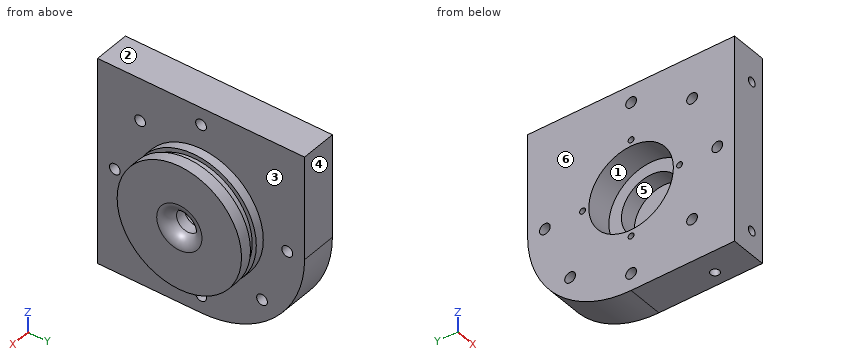
```python
from build123d import *

# Parameters (mm, degrees)
SKETCH1_R                     = 36.6395
HOUSING_FITTING_EXTRUDE_DEPTH = 16.637
HOUSING_BODY_1_DEPTH          = 21.2852
SKETCH3_R                     = 6.731
IMPELLER_BORE_DEPTH           = 17.018
SKETCH4_R                     = 4
SHAFT_BORE_DEPTH              = 20.9042
O_RING_CUT_DEPTH              = 1.27
O_RING_CUT_DEPTH_BACK         = 3.175
SKETCH5_R                     = 36.6395
SKETCH5_R_2                   = 34.2265
SKETCH12_R                    = 3.175
CUT_EXTRUDE2_DEPTH            = 21.2852
CIRPATTERN1_COUNT             = 8
SKETCH14_R                    = 2.5796875
CUT_EXTRUDE4_DEPTH            = 16.51
SKETCH15_R                    = 2.5796875
CUT_EXTRUDE5_DEPTH            = 10.922
FILLET1_R                     = 6.604
SKETCH17_R                    = 17.5006
CUT_EXTRUDE8_DEPTH            = 25.2222
SKETCH18_R                    = 24.9174
CUT_EXTRUDE9_DEPTH            = 15.3162
SKETCH19_R                    = 1.7272
CUT_EXTRUDE10_DEPTH           = 9.525


with BuildPart() as part:
    # Sketch1 → Housing Fitting Extrude (new body)
    with BuildSketch(Plane(origin=(0, 0, 0), x_dir=(0, 0, -1), z_dir=(1, 0, 0))):
        Circle(SKETCH1_R)
    extrude(amount=HOUSING_FITTING_EXTRUDE_DEPTH)

    # Sketch2 → Housing Body 1 (add)
    with BuildSketch(Plane.ZY):
        with BuildLine():
            Line((60.96, 0), (60.96, 60.96))
            Line((60.96, 60.96), (0, 60.96))
            ThreePointArc((0, 60.96), (-43.105229381, 43.105229381), (-60.96, 0))
            Line((-60.96, 0), (-60.96, -54.61))
            Line((-60.96, -54.61), (-60.96, -60.96))
            Line((-60.96, -60.96), (60.96, -60.96))
            Line((60.96, -60.96), (60.96, -54.61))
            Line((60.96, -54.61), (60.96, 0))
        make_face()
    extrude(amount=HOUSING_BODY_1_DEPTH)

    # Sketch3 → Impeller Bore (cut)
    with BuildSketch(Plane(origin=(16.637, 0, 0), x_dir=(0, 0, -1), z_dir=(1, 0, 0))):
        Circle(SKETCH3_R)
    extrude(amount=-IMPELLER_BORE_DEPTH, mode=Mode.SUBTRACT)

    # Sketch4 → Shaft Bore (cut)
    with BuildSketch(Plane(origin=(-0.381, 0, 0), x_dir=(0, 0, -1), z_dir=(1, 0, 0))):
        Circle(SKETCH4_R)
    extrude(amount=-SHAFT_BORE_DEPTH, mode=Mode.SUBTRACT)

    # Sketch5 → O-Ring Cut (cut, two sides: drawn at the far end of the back side and taken through both)
    with BuildSketch(Plane(origin=(8.509, 0, 0), x_dir=(0, 0, -1), z_dir=(1, 0, 0)).offset(-O_RING_CUT_DEPTH_BACK)):
        Circle(SKETCH5_R)
        Circle(SKETCH5_R_2, mode=Mode.SUBTRACT)
    extrude(amount=O_RING_CUT_DEPTH + O_RING_CUT_DEPTH_BACK, mode=Mode.SUBTRACT)

    # Sketch12 → Cut-Extrude2 (cut)
    with BuildSketch(Plane(origin=(0, 0, 0), x_dir=(0, 0, -1), z_dir=(1, 0, 0))):
        with Locations((-50.8, 0)):
            Circle(SKETCH12_R)
    cut_extrude2 = extrude(amount=-CUT_EXTRUDE2_DEPTH, mode=Mode.SUBTRACT)

    # CirPattern1: Cut-Extrude2 ×8 about axis, 1 skipped
    cirpattern1_axis = Axis((0, 0, 0), (1, 0, 0))
    add([cut_extrude2.rotate(cirpattern1_axis, i * 360 / CIRPATTERN1_COUNT) for i in range(1, CIRPATTERN1_COUNT) if i not in (7,)], mode=Mode.SUBTRACT)

    # Sketch14 → Cut-Extrude4 (cut)
    with BuildSketch(Plane.XZ.offset(60.96)):
        with Locations(Location((-8.128, -46.754349092, 0), (0, 0, 270))):
            Circle(SKETCH14_R)
        with Locations(Location((-8.128, 41.914080666, 0), (0, 0, 270))):
            Circle(SKETCH14_R)
    extrude(amount=-CUT_EXTRUDE4_DEPTH, mode=Mode.SUBTRACT)

    # Sketch15 → Cut-Extrude5 (cut)
    with BuildSketch(Plane(origin=(0, 0, -60.96), x_dir=(-1, 0, 0), z_dir=(0, 0, -1))):
        with Locations(Location((8.128, -39.337514031, 0), (0, 0, 90))):
            Circle(SKETCH15_R)
    extrude(amount=-CUT_EXTRUDE5_DEPTH, mode=Mode.SUBTRACT)

    # Fillet1
    fillet1_edges = [part.edges().sort_by_distance(p)[0] for p in [
        (16.637, 0, 6.731),
    ]]
    fillet(fillet1_edges, radius=FILLET1_R)

    # Sketch17 → Cut-Extrude8 (cut)
    with BuildSketch(Plane.ZY.offset(21.2852)):
        Circle(SKETCH17_R)
    extrude(amount=-CUT_EXTRUDE8_DEPTH, mode=Mode.SUBTRACT)

    # Sketch18 → Cut-Extrude9 (cut)
    with BuildSketch(Plane.ZY.offset(21.2852)):
        Circle(SKETCH18_R)
    extrude(amount=-CUT_EXTRUDE9_DEPTH, mode=Mode.SUBTRACT)

    # Sketch19 → Cut-Extrude10 (cut)
    with BuildSketch(Plane.ZY.offset(21.2852)):
        with Locations((0, 28.575)):
            Circle(SKETCH19_R)
        with Locations((28.575, 0)):
            Circle(SKETCH19_R)
        with Locations((0, -28.575)):
            Circle(SKETCH19_R)
        with Locations((-28.575, 0)):
            Circle(SKETCH19_R)
    extrude(amount=-CUT_EXTRUDE10_DEPTH, mode=Mode.SUBTRACT)


solid = part.part
```
Geometry: final body of the model. Coordinates: model frame, mm. Face numbers are marked on the shaded views. A direction names the side the tool comes from. Round coordinates to 2 decimals unless told otherwise and drop trailing zeros. Order: outer loops, then holes, each group sorted by start corner. A loop starts at its lowest first (then second) coordinate and runs counter-clockwise, first axis right, second up. Notation, with made-up numbers: M 37,-6.5 L 86,-6.5 A11 ccw 86,7.5 Z; hole C 89,84.25 d10. An arc over 180 degrees is marked long. Use one line per item in the form item = value. Start each with the question number.
Q1. Material intervals for line 1 (Y direction, x = 6.25, z = 0); line 2 (Y direction, x = -9, z = 50.5); line 3 (Y direction, x = -13.5, z = 2), sorted ascending. Write a range as [from, to].
Q2. Pin query (flat end, axial travel): pin 1 Ø2 at (x, y) = (10.5, -26) entering from +Z; pin 2 Ø1.5 at (y, z) = (-29, -27) entering from +X; pin 3 Ø21.5 at (y, z) = (0, 0) entering from +X. Return the tip coordinate at first contact, or that it passes through.
Q3. Cut plane A-A (z = 50.8). Return loops of the section in (x, y) (3 decimals).
Q4. Cut plane C-C (y = 50.8). Return loops of the section in (x, z) (3 decimals).
Q5. Access query for the marked faces 1, 2 and 3. Directions: +Z, -Z, +X, -X, +Y, -Y. A direction counts if a zero-diameter tool reaches every point of the face in a straight line with its end or side. Return the directions, or none.
Q6. Cut plane B-B (y = -49.5). Return loops of the section in (x, z), and give its area (3 significant figures).
Q7. Cut plane D-D (y = 22). Return loops of the section in (x, z), and give its area (3 significant figures).
Q8. Mould query, pull axis Y, two halves, no side actions, for the marked faces 4, 5 and 6. Classes: +Y half, -Y half, draft (parallel to the pull), parting line (faces both ways), or undercut.
Geometry results:
q1.line_1 = [-34.23, -6.73], [6.73, 34.23]
q1.line_2 = [-60.96, -3.16], [3.16, 60.96]
q1.line_3 = [-60.96, -53.27], [-48.33, -24.84], [24.84, 48.33], [53.27, 60.96]
q2.pin_1 = 26.79
q2.pin_2 = 0
q2.pin_3 = 16.11
q3.outline = M -21.285,-60.96 L 0,-60.96 L 0,-3.175 L -21.285,-3.175 Z; M -21.285,3.175 L 0,3.175 L 0,60.96 L -21.285,60.96 Z
q4.outline = M -21.285,-33.697 L 0,-33.697 L 0,-3.175 L -21.285,-3.175 Z; M -21.285,3.175 L 0,3.175 L 0,60.96 L -21.285,60.96 Z
q5.face_1 = -X
q5.face_2 = +Z, +X, -X, +Y, -Y
q5.face_3 = +X
q6.outline = M -21.29,-60.96 L 0,-60.96 L 0,-2.9 L -21.29,-2.9 Z; M -21.29,2.9 L 0,2.9 L 0,60.96 L -21.29,60.96 Z; hole C -8.13,-46.75 d5.16; hole C -8.13,41.91 d5.16
q6.area = 2,430 mm^2
q7.outline = M -21.29,-56.85 L 0,-56.85 L 0,-29.3 L 5.33,-29.3 L 5.33,-26.22 L 9.78,-26.22 L 9.78,-29.3 L 16.64,-29.3 L 16.64,29.3 L 9.78,29.3 L 9.78,26.22 L 5.33,26.22 L 5.33,29.3 L 0,29.3 L 0,60.96 L -21.29,60.96 L -21.29,11.7 L -5.97,11.7 L -5.97,-11.7 L -21.29,-11.7 Z
q7.area = 3,100 mm^2
q8.face_4 = +Y half
q8.face_5 = undercut
q8.face_6 = draft
